```python
from build123d import *

# Parameters (mm, degrees)
F0_W     = 35
F0_H     = 40
F1_DEPTH = 4
F2_R     = 5
F3_R     = 3.75
F4_DEPTH = 2
F5_R     = 2
F6_DEPTH = 5
F7_R     = 2
F8_DEPTH = 5


with BuildPart() as f1:
    # F0 (on Top) → F1 (new body)
    with BuildSketch(Plane.XY):
        with Locations((-15.016379, 5.064304)):
            Rectangle(F0_W, F0_H)
    extrude(amount=F1_DEPTH)

    # F2
    f2_edges = [f1.edges().sort_by_distance(p)[0] for p in [
        (-32.516379, 25.064304, 2),
        (-32.516379, -14.935696, 2),
    ]]
    fillet(f2_edges, radius=F2_R)

    # F3 (on face) → F4 (cut)
    with BuildSketch(Plane.XY.offset(4)):
        with Locations((-17.516379, -4.935696)):
            Circle(F3_R)
        with Locations((-17.516379, 15.064304)):
            Circle(F3_R)
    extrude(amount=-F4_DEPTH, mode=Mode.SUBTRACT)

    # F5 (on face) → F6 (cut)
    with BuildSketch(Plane.XY.offset(2)):
        with Locations((-17.516379, 15.064304)):
            Circle(F5_R)
    extrude(amount=-F6_DEPTH, mode=Mode.SUBTRACT)

    # F7 (on face) → F8 (cut)
    with BuildSketch(Plane.XY.offset(2)):
        with Locations((-17.516379, -4.935696)):
            Circle(F7_R)
    extrude(amount=-F8_DEPTH, mode=Mode.SUBTRACT)

    # F9: F1 across face


with BuildPart() as f1_1:
    add(f1.part)
    add(f1.part.mirror(Plane(origin=(2.483621, 5.064304, 2), x_dir=(0, 1, 0), z_dir=(1, 0, 0))))


solid = f1_1.part
```
Here's how the part is built. I have some questions about the finished solid (model axes, mm). A direction names the side the tool comes from. Round coordinates to 2 decimals unless told otherwise and drop trailing zeros. Order: outer loops, then holes, each group sorted by start corner. A loop starts at its lowest first (then second) coordinate and runs counter-clockwise, first axis right, second up. Notation, with made-up numbers: (36.25, -20.75) -> (81.25, -20.75) arc R27 cw to (81.25, 11.25) -> close; hole circle Ø7 at (6, -21). An arc over 180 degrees is marked (long way). Use a Markdown table: item, result. Add a question column.
(1) For pin 1 Ø6 at (x, y) = (22.48, 15.06) entering from +Z, with a flat end and sliding along its axis, tell me the tip position at first contact or that it passes through.
(2) For faces 1 (the face through (-16, -7, 2)), 2 (the face through (-15.61, -4.33, 1.01)), which set-ups out of +Z, -Z, +X, -X, +Y, -Y let a thin tool reach every point of the face, with its end or its side?
(3) If we mould it in two halves opening along Y, with no side actions, what happens to faces 3 (the face through (36.06, -13.43, 2.03)), 4 (the face through (-31.09, 23.56, 2.03)), 5 (the face through (20.576, 15.665, 1.014)), 6 (the face through (18.907, 16.191, 3.014))? For each: released by +Y, released by -Y, zero draft, split by the parting line, or undercut.
(4) I need wall thicknesses on line 1 along Y through (x, z) = (-19, 2.7); line 2 along X through (y, z) = (16.5, 3.35); line 3 along X through (y, z) = (18, 2.3). Which ranges of each line are inside material? Lowest first, please.
(5) Suppose I cut it at B-B, the plane z = 0.7. Please give me the cut outline in (x, y).
(6) Suppose I cut it at C-C, the plane y = -4. Please give me the cut outline in (x, z) (3 decimals), and give its area (3 significant figures).
(7) Suppose I cut it at A-A, the plane x = -18. Please give me the cut outline in (y, z).
(8) Suppose I cut it at D-D, the plane y = 23.5. Please give me the cut outline in (x, z), and give its area (3 significant figures).
Verdict:
| question | item | result |
|---|---|---|
| 1 | pin 1 | z = 2 |
| 2 | face 1 | +Z |
| 2 | face 2 | +Z, -Z |
| 3 | face 3 | released by -Y |
| 3 | face 4 | released by +Y |
| 3 | face 5 | undercut |
| 3 | face 6 | undercut |
| 4 | line 1 | -14.94 to -8.38, -1.49 to 11.62, 18.51 to 25.06 |
| 4 | line 2 | -32.52 to -20.98, -14.05 to 19.02, 25.95 to 37.48 |
| 4 | line 3 | -32.52 to -19.85, -15.18 to 20.15, 24.82 to 37.48 |
| 5 | outline | (-32.52, -9.94) arc R5 ccw to (-27.52, -14.94) -> (32.48, -14.94) arc R5 ccw to (37.48, -9.94) -> (37.48, 20.06) arc R5 ccw to (32.48, 25.06) -> (-27.52, 25.06) arc R5 ccw to (-32.52, 20.06) -> close; hole circle Ø4 at (-17.52, -4.94); hole circle Ø4 at (-17.52, 15.06); hole circle Ø4 at (22.48, -4.94); hole circle Ø4 at (22.48, 15.06) |
| 6 | outline | (-32.516, 0) -> (-19.284, 0) -> (-19.284, 2) -> (-21.148, 2) -> (-21.148, 4) -> (-32.516, 4) -> close; (-15.749, 0) -> (20.716, 0) -> (20.716, 2) -> (18.852, 2) -> (18.852, 4) -> (-13.885, 4) -> (-13.885, 2) -> (-15.749, 2) -> close; (24.251, 0) -> (37.484, 0) -> (37.484, 4) -> (26.115, 4) -> (26.115, 2) -> (24.251, 2) -> close |
| 6 | area | 237 mm2 |
| 7 | outline | (-14.94, 0) -> (-6.88, 0) -> (-6.88, 2) -> (-8.65, 2) -> (-8.65, 4) -> (-14.94, 4) -> close; (-3, 0) -> (13.12, 0) -> (13.12, 2) -> (11.35, 2) -> (11.35, 4) -> (-1.22, 4) -> (-1.22, 2) -> (-3, 2) -> close; (17, 0) -> (25.06, 0) -> (25.06, 4) -> (18.78, 4) -> (18.78, 2) -> (17, 2) -> close |
| 8 | outline | (-31.15, 0) -> (36.12, 0) -> (36.12, 4) -> (-31.15, 4) -> close |
| 8 | area | 269 mm2 |
